```python
from build123d import *

# Parameters (mm, degrees)
F0_W      = 16.51
F0_H      = 15.24
F1_DEPTH  = 1.4986
F2_R      = 1.27
F3_DEPTH  = 1.4986
F4_R      = 2.54
F5_W      = 5.8166
F5_H      = 7.8994
F6_DEPTH  = 5.334
F7_W      = 6.3754
F7_H      = 3.81
F7_W_2    = 0.508
F7_H_2    = 0.508
F8_DEPTH  = 5.0546
F9_W      = 3.8771615364
F9_H      = 0.762
F10_DEPTH = 1.27
F11_R     = 0.4064
F12_DEPTH = 1.4986
F13_W     = 0.9398
F13_H     = 1.8542
F14_DEPTH = 1.3208


with BuildPart() as f1:
    # F0 (on Top) → F1 (new body)
    with BuildSketch(Plane.XY):
        Rectangle(F0_W, F0_H)
    extrude(amount=F1_DEPTH)

    # F2 (on face) → F3 (cut, through all)
    with BuildSketch(Plane.XY.offset(1.4986)):
        with Locations((5.715, 5.08)):
            Circle(F2_R)
    extrude(amount=-F3_DEPTH, mode=Mode.SUBTRACT)

    # F4
    f4_edges = [f1.edges().sort_by_distance(p)[0] for p in [
        (8.255, -7.62, 0.7493),
        (8.255, 7.62, 0.7493),
        (-8.255, -7.62, 0.7493),
        (-8.255, 7.62, 0.7493),
    ]]
    fillet(f4_edges, radius=F4_R)

    # F5 (on face) → F6 (join)
    with BuildSketch(Plane.XY.offset(1.4986)):
        with Locations((5.3467, -1.524)):
            Rectangle(F5_W, F5_H)
    extrude(amount=F6_DEPTH)

    # F7 (on face) → F8 (cut, through all)
    with BuildSketch(Plane.YZ.offset(8.255)):
        with Locations((-1.524, 4.1656)):
            Rectangle(F7_W, F7_H)
        with Locations((-2.794, 4.1656)):
            Rectangle(F7_W_2, F7_H_2, mode=Mode.SUBTRACT)
        with Locations((-0.254, 4.1656)):
            Rectangle(F7_W_2, F7_H_2, mode=Mode.SUBTRACT)
    extrude(amount=-F8_DEPTH, mode=Mode.SUBTRACT)

    # F9 (on face) → F10 (cut)
    with BuildSketch(Plane.XY.offset(6.8326)):
        with Locations((4.3769807682, 0.508)):
            Rectangle(F9_W, F9_H)
        with Locations((4.3769807682, -3.556)):
            Rectangle(F9_W, F9_H)
    extrude(amount=-F10_DEPTH, mode=Mode.SUBTRACT)

    # F11 (on face) → F12 (cut, through all)
    with BuildSketch(Plane.XY.offset(1.4986)):
        with Locations((-6.4262, 6.3246)):
            Circle(F11_R)
        with Locations((-3.8862, 6.3246)):
            Circle(F11_R)
        with Locations((-1.3462, 6.3246)):
            Circle(F11_R)
    extrude(amount=-F12_DEPTH, mode=Mode.SUBTRACT)

    # F13 (on face) → F14 (join)
    with BuildSketch(Plane.XY.offset(1.4986)):
        with Locations((-6.0639006243, 1.7056578491)):
            Rectangle(F13_W, F13_H)
        with Locations((-4.4129006243, 1.7056578491)):
            Rectangle(F13_W, F13_H)
        with Locations((-2.7619006243, 1.7056578491)):
            Rectangle(F13_W, F13_H)
        with Locations((-1.1109006243, 1.7056578491)):
            Rectangle(F13_W, F13_H)
        with Locations((-6.0639006243, -1.7056578491)):
            Rectangle(F13_W, F13_H)
        with Locations((-1.1109006243, -1.7056578491)):
            Rectangle(F13_W, F13_H)
        with Locations((-4.4129006243, -1.7056578491)):
            Rectangle(F13_W, F13_H)
        with Locations((-2.7619006243, -1.7056578491)):
            Rectangle(F13_W, F13_H)
    extrude(amount=F14_DEPTH)


solid = f1.part
```
Can you work these out from the model? Positions are in its coordinate system, mm. A direction names the side the tool comes from. Round coordinates to 2 decimals unless told otherwise and drop trailing zeros. Loops run counter-clockwise (first coordinate to the right, second up) from the corner with the lowest first, then second, coordinate; pieces in that order, holes last. Notation, with made-up numbers: M 60,-0.75 L 98,-0.75 A34 cw 98,33.25 Z; hole C 51,-3 d10. An arc over 180 degrees is marked long. Answer as a JSON object with one key per item and string values. Group by question number.
Q1. Please list where these lines run through material, in increasing order: L1, parallel to X at y = -1.25, z = 2.5; L2, parallel to X at y = 6, z = 0.5; L3, parallel to Y at x = 6, z = 3.
Q2. Will these pins go through, and if not, where does the flat tip stop? pin 1 (1 mm diameter, centred on x = -4.5, z = 2.5, fed in from -Y); pin 2 (1.6 mm diameter, centred on x = 5, z = 3.5, fed in from +Y); pin 3 (0.6 mm diameter, centred on x = 3, y = 0.5, fed in from +Z).
Q3. Imagine slicing it at B-B, the plane z = 5. Please give me the cut outline in (x, y) (3 decimals).
Q4. On a 3-axis mill with a long thin cutter (end or side, diameter ignored), from which of +Z, -Z, +X, -X, +Y, -Y can I reach the whole of each face in a straight line? I mean faces 1 (the flat face through (3.9, 0.127, 6.3)), 2 (the flat face through (-4.4, 1.7, 2.819)), 3 (the flat face through (6, 1.664, 4)). Say none if no direction works.
Q5. We'd pull the mould along Y, two halves only. Please class faces 4 (the flat face through (-0.641, 2, 2)), 5 (the flat face through (6, -2, 6.071)), 6 (the flat face through (-4.4, -2.633, 2.1)): +Y half, -Y half, draft (parallel to the pull), parting line (faces both ways), or undercut.
Q6. Imagine slicing it at C-C, the plane x = 5. Count the separate pieces of the cut face and the enclosed holes in it, then the cut area to 3 significant figures.
Q7. Imagine slicing it at A-A, the plane y = -3.5. Please give me the cut outline in (x, z) (3 decimals), then the cut area to 3 significant figures.
Findings:
{
 "1": {"L1": "x = -6.53 to -5.59, -4.88 to -3.94, -3.23 to -2.29, -1.58 to -0.64, 2.44 to 3.2", "L2": "x = -8.08 to -6.67, -6.18 to -4.13, -3.64 to -1.59, -1.1 to 4.84, 6.59 to 8.08", "L3": "y = -5.47 to -4.71, 1.66 to 2.43"},
 "2": {"pin 1": "stops at y = -2.63", "pin 2": "stops at y = 2.43", "pin 3": "stops at z = 5.56"},
 "3": {"outline": "M 2.438,-5.474 L 8.255,-5.474 L 8.255,-4.712 L 3.2,-4.712 L 3.2,1.664 L 8.255,1.664 L 8.255,2.426 L 2.438,2.426 Z"},
 "4": {"face 1": "+Z, -X", "face 2": "+Z, -X, +Y, -Y", "face 3": "+X"},
 "5": {"face 4": "draft", "face 5": "undercut", "face 6": "-Y half"},
 "6": {"separate pieces": "5", "enclosed holes": "0", "area": "36.9 mm2"},
 "7": {"outline": "M -8.255,0 L 8.255,0 L 8.255,2.261 L 3.2,2.261 L 3.2,5.563 L 2.438,5.563 L 2.438,1.499 L -8.255,1.499 Z; M 6.316,6.071 L 8.255,6.071 L 8.255,6.833 L 6.316,6.833 Z", "area": "33.2 mm2"}
}
